Check sheet for the modelled part. Datum: model origin and axes. Units: mm. A direction names the side the tool comes from. Coordinates: 2 decimals unless noted, no trailing zeros. Loops run counter-clockwise (first coordinate to the right, second up) from the corner with the lowest first, then second, coordinate; pieces in that order, holes last. Notation, with made-up numbers: M 13,56.5 L 23,56.5 A10 cw 23,60.5 Z; hole C 68.25,6.5 d6. An arc over 180 degrees is marked long. Use CSV: the item, a comma, the result in double quotes. Start each with the question number.
(1) Draft check along Z on faces 1 (the cylindrical face through (-1.71, 2.19, -0.38)), 2 (the flat face through (0, 2.8, 0)), 3 (the flat face through (0, 0, 0)). Enter one of: pulls with the +Z half, pulls with the -Z half, needs draft (parallel to the pull), parting line crosses it, or undercut.
(2) Section check D-D on y = 0.25. Record the cut outline in (x, z), and give its area (3 significant figures).
(3) Set-up check for faces 4 (the cylindrical face through (-2.685, 0.592, -0.596)), 5 (the flat face through (0, 1.2, 2)): record each of +Z, -Z, +X, -X, +Y, -Y from which the full face is reachable in a straight line by a thin tool's end or side.
(4) Section check B-B on x = 0. Record the cut outline in (y, z), and give its area (3 significant figures).
(5) Section check C-C on y = -5. Record the cut outline in (x, z), and give its area (3 significant figures).
(6) Section check A-A on z = 0. Record the cut outline in (x, y), and give its area (3 significant figures).
(7) Scan lines: line 1 (X direction, y = 3, z = 0); line 2 (Y direction, x = 0.9, z = -0.35); line 3 (Y direction, x = -1.9, z = -1.1). Record each from-to range of solid material in increasing order.
(8) Go/stop test with flat-tipped pins: pin 1 Ø1 at (y, z) = (-1.5, -1) entering from +X; pin 2 Ø1 at (y, z) = (0, -1.5) entering from +X; pin 3 Ø1.2 at (x, z) = (0, 0) entering from -Y. Record where each tip stops, or that it passes through.
from build123d import *

# Parameters (mm, degrees)
SKETCH1_R           = 2.75
BOSS_EXTRUDE1_DEPTH = 1.2
SKETCH2_R           = 1.75
BOSS_EXTRUDE2_DEPTH = 2
SKETCH3_R           = 0.736254348
CUT_EXTRUDE1_DEPTH  = 0.4
SKETCH4_R           = 0.143122077
BOSS_EXTRUDE3_DEPTH = 5.4


with BuildPart() as part:
    # Sketch1 → Boss-Extrude1 (new body)
    with BuildSketch(Plane(origin=(0, 0, 0), x_dir=(1, 0, 0), z_dir=(0, 1, 0))):
        with Locations(Location((0, 0, 0), (0, 0, 270))):
            Circle(SKETCH1_R)
    extrude(amount=BOSS_EXTRUDE1_DEPTH)

    # Sketch2 → Boss-Extrude2 (add)
    with BuildSketch(Plane(origin=(0, 1.2, 0), x_dir=(1, 0, 0), z_dir=(0, 1, 0))):
        with Locations(Location((0, 0, 0), (0, 0, 270))):
            Circle(SKETCH2_R)
    extrude(amount=BOSS_EXTRUDE2_DEPTH)

    # Sketch3 → Cut-Extrude1 (cut)
    with BuildSketch(Plane(origin=(0, 3.2, 0), x_dir=(1, 0, 0), z_dir=(0, 1, 0))):
        with Locations(Location((0, 0, 0), (0, 0, 270))):
            Circle(SKETCH3_R)
    extrude(amount=-CUT_EXTRUDE1_DEPTH, mode=Mode.SUBTRACT)

    # Sketch4 → Boss-Extrude3 (add)
    with BuildSketch(Plane.XZ):
        with Locations(Location((0, 1.733276442, 0), (0, 0, 90))):
            Circle(SKETCH4_R)
        with Locations(Location((1.501061431, -0.866638221, 0), (0, 0, 90))):
            Circle(SKETCH4_R)
        with Locations(Location((-1.501061431, -0.866638221, 0), (0, 0, 90))):
            Circle(SKETCH4_R)
    extrude(amount=BOSS_EXTRUDE3_DEPTH)


solid = part.part
Outcome:
1,face 1,"parting line crosses it"
1,face 2,"undercut"
1,face 3,"needs draft"
2,outline,"C 0,0 d5.5"
2,area,"23.8 mm²"
3,face 4,"+Y, -Y"
3,face 5,"+Y"
4,outline,"M -5.4,1.59 L 0,1.59 L 0,-2.75 L 1.2,-2.75 L 1.2,-1.75 L 3.2,-1.75 L 3.2,-0.74 L 2.8,-0.74 L 2.8,0.74 L 3.2,0.74 L 3.2,1.75 L 1.2,1.75 L 1.2,2.75 L 0,2.75 L 0,1.88 L -5.4,1.88 Z"
4,area,"14.6 mm²"
5,outline,"C -1.5,-0.87 d0.29; C 0,1.73 d0.29; C 1.5,-0.87 d0.29"
5,area,"0.193 mm²"
6,outline,"M -2.75,0 L 2.75,0 L 2.75,1.2 L 1.75,1.2 L 1.75,3.2 L 0.74,3.2 L 0.74,2.8 L -0.74,2.8 L -0.74,3.2 L -1.75,3.2 L -1.75,1.2 L -2.75,1.2 Z"
6,area,"13.0 mm²"
7,line 1,"x = -1.75 to -0.74, 0.74 to 1.75"
7,line 2,"y = 0 to 3.2"
7,line 3,"y = 0 to 1.2"
8,pin 1,"stops at x = 1.64"
8,pin 2,"stops at x = 2.56"
8,pin 3,"stops at y = 0"
